Input: part model. Units: mm. Frame: model coordinates. A direction names the side the tool comes from. Coordinates: 2 decimals unless noted, no trailing zeros. Write each loop counter-clockwise with the first axis right and the second up, starting at its lowest first coordinate (ties: lowest second). Pieces come first, ordered by that corner, then holes. Notation, with made-up numbers: (-7, -22.5) - (41, -22.5) arc R25 ccw to (41, -4.5) - close; hole circle Ø3 at (-39.75, 81.25). An arc over 180 degrees is marked (long way). One line per question, with ' | ' between items. Start each with the question number.
1) Section query A-A on z = 85. Return loops of the section in (x, y), and give its area (3 significant figures).
2) Draft query along Z for faces 6 (the flat face through (4, 0, 86.36)), 7 (the flat face through (-4, 0, 88.9)), 8 (the flat face through (5.08, 0, 88)). Return one class per face: released by +Z, released by -Z, zero draft, split by the parting line, or undercut.
3) Section query B-B on z = 37. Return loops of the section in (x, y), and give its area (3 significant figures).
4) Section query C-C on z = 66.5. Return loops of the section in (x, y), and give its area (3 significant figures).
5) First-contact query: P1, Ø8, axis at y = -16.5, z = 41.5, coming from the +X side; P2, Ø1.3, axis at x = 4, y = -1, coming from the +Z side; P3, Ø1.3, axis at y = 1, z = 85.5, coming from the -X side; P4, Ø4, axis at x = 1, z = 86, coming from the -Y side. Flat tips, straight axial feed; report the tip coordinate or a pass-through.
6) Line query: line 1 (Z direction, x = 6.5, y = 3); line 2 (Z direction, x = -2.5, y = -13.5); line 3 (Y direction, x = -4.5, z = 47). Output: solid intervals per line, ascending.
7) Reachability of faces 1 (the flat face through (-5.08, 0, 88)), 2 (the flat face through (0, -2.54, 88)), 3 (the flat face through (-9, 8, 18.953)), 4 (the flat face through (2.54, 0, 85)), 5 (the flat face through (-4, 0, 86.36)) from +Z, -Z, +X, -X, +Y, -Y: full face, straight path, thin tool, end or side. Return the list, or none.
```python
from build123d import *

# Parameters (mm, degrees)
F2_W     = 5.08
F2_H     = 5.08
F3_DEPTH = 2.54
F4_W     = 2.54
F4_H     = 5.08
F4_W_2   = 5.08
F5_DEPTH = 2.54
F6_W     = 5.08
F6_H     = 5.08
F7_DEPTH = 2.54
F8_R     = 1.27


with BuildPart() as f1:
    # F0 (on Front) → F1 (revolve)
    with BuildSketch(Plane.XZ):
        with BuildLine():
            Line((0, 83.82), (0, 0))
            Line((0, 0), (22.86, 0))
            Line((22.86, 0), (22.86, 5.08))
            ThreePointArc((22.86, 5.08), (16.6236237238, 10.7941273506), (14.3945977767, 18.9534829479))
            Line((14.3945977767, 18.9534829479), (11.8545977767, 18.9534829479))
            ThreePointArc((11.8545977767, 18.9534829479), (8.4999635218, 43.2049976701), (7.62, 67.6716116881))
            Line((7.62, 67.6716116881), (11.43, 67.6716116881))
            ThreePointArc((11.43, 67.6716116881), (12.7, 68.9416116881), (11.43, 70.2116116881))
            Line((11.43, 70.2116116881), (7.62, 70.2116116881))
            Line((7.62, 70.2116116881), (12.7, 83.82))
            Line((12.7, 83.82), (0, 83.82))
        make_face()
    revolve(axis=Axis((0, 0, 41.91), (0, 0, 1)))

    # F2 (on face) → F3 (join)
    with BuildSketch(Plane.XY.offset(83.82)):
        Rectangle(F2_W, F2_H)
    extrude(amount=F3_DEPTH)

    # F4 (on face) → F5 (join)
    with BuildSketch(Plane.XY.offset(86.36)):
        with Locations((-3.81, 0)):
            Rectangle(F4_W, F4_H)
        Rectangle(F4_W_2, F4_H)
        with Locations((3.81, 0)):
            Rectangle(F4_W, F4_H)
    extrude(amount=F5_DEPTH)

    # F6 (on face) → F7 (join)
    with BuildSketch(Plane.XY.offset(88.9)):
        Rectangle(F6_W, F6_H)
    extrude(amount=F7_DEPTH)

    # F8
    f8_edges = [f1.edges().sort_by_distance(p)[0] for p in [
        (-14.394598, 0, 18.953483),
    ]]
    fillet(f8_edges, radius=F8_R)


solid = f1.part
```
Answer key:
1) outline: (-2.54, -2.54) - (2.54, -2.54) - (2.54, 2.54) - (-2.54, 2.54) - close | area: 25.8 mm²
2) face 6: undercut | face 7: released by +Z | face 8: zero draft
3) outline: circle Ø18.24 at (0, 0) | area: 261 mm²
4) outline: circle Ø15.21 at (0, 0) | area: 182 mm²
5) P1: through | P2: z = 88.9 | P3: x = -2.54 | P4: y = -2.54
6) line 1: 0 to 83.82 | line 2: 0 to 18.82 | line 3: -6.86 to 6.86
7) face 1: +Z, -X, +Y, -Y | face 2: +Z, +X, -X, -Y | face 3: none | face 4: +X, +Y, -Y | face 5: -X, +Y, -Y
